```python
from build123d import *

# Parameters (mm, degrees)
ESBO_O1_W                                            = 10
ESBO_O1_H                                            = 11.5
RESSALTO_EXTRUS_O1_DEPTH                             = 9
ESBO_O2_W                                            = 4
ESBO_O2_H                                            = 0.85
CORTE_EXTRUS_O1_DEPTH                                = 10
ESBO_O3_W                                            = 3
ESBO_O3_H                                            = 1.6
RESSALTO_EXTRUS_O2_DEPTH                             = 1
ESBO_O4_W                                            = 3
ESBO_O4_H                                            = 1.6
RESSALTO_EXTRUS_O3_DEPTH                             = 1
ESBO_O5_W                                            = 4
ESBO_O5_H                                            = 1.5
CORTE_EXTRUS_O2_DEPTH                                = 11
ESBO_O6_W                                            = 1.5
ESBO_O6_H                                            = 1
RESSALTO_EXTRUS_O4_DEPTH                             = 1
ESBO_O7_W                                            = 1.5
ESBO_O7_H                                            = 1.5
CORTE_EXTRUS_O3_DEPTH                                = 6
ESBO_O8_W                                            = 1.5
ESBO_O8_H                                            = 1
RESSALTO_EXTRUS_O5_DEPTH                             = 1
ESBO_O9_W                                            = 1.5
ESBO_O9_H                                            = 1.5
CORTE_EXTRUS_O4_DEPTH                                = 6
ESBO_O10_W                                           = 1.5
ESBO_O10_H                                           = 1.5
RESSALTO_EXTRUS_O6_DEPTH                             = 1.5
ESBO_O11_W                                           = 1.5
ESBO_O11_H                                           = 1.5
RESSALTO_EXTRUS_O7_DEPTH                             = 1.5
ESBO_O12_W                                           = 9.5
ESBO_O12_H                                           = 4.15
REBAIXO_PARA_PARAFUSO_DE_M_QUINA_DE_CABE_D           = 3.3
REBAIXO_PARA_PARAFUSO_DE_M_QUINA_DE_CABE_DEPTH       = 9.5
REBAIXO_PARA_PARAFUSO_DE_M_QUINA_DE_CABE_CBORE_D     = 6
REBAIXO_PARA_PARAFUSO_DE_M_QUINA_DE_CABE_CBORE_DEPTH = 0.375
FILETE1_R                                            = 1
RESSALTO_EXTRUS_O9_DEPTH                             = 0.2


with BuildPart() as part:
    # Esboço1 → Ressalto-extrusão1 (new body)
    with BuildSketch(Plane(origin=(10, 0, 0), x_dir=(0, 0, -1), z_dir=(1, 0, 0))):
        with Locations((0, -0.75)):
            Rectangle(ESBO_O1_W, ESBO_O1_H)
    extrude(amount=-RESSALTO_EXTRUS_O1_DEPTH)

    # Esboço2 → Corte-extrusão1 (cut, through all)
    with BuildSketch(Plane(origin=(10, 0, 0), x_dir=(0, 0, -1), z_dir=(1, 0, 0))):
        with Locations((0, 4.575)):
            Rectangle(ESBO_O2_W, ESBO_O2_H)
    extrude(amount=-CORTE_EXTRUS_O1_DEPTH, mode=Mode.SUBTRACT)

    # Esboço3 → Ressalto-extrusão2 (add)
    with BuildSketch(Plane.ZY.offset(-1)):
        with Locations((3.5, 4.2)):
            Rectangle(ESBO_O3_W, ESBO_O3_H)
    extrude(amount=RESSALTO_EXTRUS_O2_DEPTH)

    # Esboço4 → Ressalto-extrusão3 (add)
    with BuildSketch(Plane.ZY.offset(-1)):
        with Locations((-3.5, 4.2)):
            Rectangle(ESBO_O4_W, ESBO_O4_H)
    extrude(amount=RESSALTO_EXTRUS_O3_DEPTH)

    # Esboço5 → Corte-extrusão2 (cut, through all)
    with BuildSketch(Plane(origin=(10, 0, 0), x_dir=(0, 0, -1), z_dir=(1, 0, 0))):
        with Locations((0, -5.75)):
            Rectangle(ESBO_O5_W, ESBO_O5_H)
    extrude(amount=-CORTE_EXTRUS_O2_DEPTH, mode=Mode.SUBTRACT)

    # Esboço6 → Ressalto-extrusão4 (add)
    with BuildSketch(Plane.ZY.offset(-1)):
        with Locations((2.75, -6)):
            Rectangle(ESBO_O6_W, ESBO_O6_H)
    extrude(amount=RESSALTO_EXTRUS_O4_DEPTH)

    # Esboço7 → Corte-extrusão3 (cut)
    with BuildSketch(Plane.ZY.offset(-1)):
        with Locations((4.25, -5.75)):
            Rectangle(ESBO_O7_W, ESBO_O7_H)
    extrude(amount=-CORTE_EXTRUS_O3_DEPTH, mode=Mode.SUBTRACT)

    # Esboço8 → Ressalto-extrusão5 (add)
    with BuildSketch(Plane.ZY.offset(-1)):
        with Locations((-2.75, -6)):
            Rectangle(ESBO_O8_W, ESBO_O8_H)
    extrude(amount=RESSALTO_EXTRUS_O5_DEPTH)

    # Esboço9 → Corte-extrusão4 (cut)
    with BuildSketch(Plane.ZY.offset(-1)):
        with Locations((-4.25, -5.75)):
            Rectangle(ESBO_O9_W, ESBO_O9_H)
    extrude(amount=-CORTE_EXTRUS_O4_DEPTH, mode=Mode.SUBTRACT)

    # Esboço10 → Ressalto-extrusão6 (add)
    with BuildSketch(Plane.XZ.offset(6.5)):
        with Locations((9.25, 4.25)):
            Rectangle(ESBO_O10_W, ESBO_O10_H)
    extrude(amount=RESSALTO_EXTRUS_O6_DEPTH)

    # Esboço11 → Ressalto-extrusão7 (add)
    with BuildSketch(Plane.XZ.offset(6.5)):
        with Locations((9.25, -4.25)):
            Rectangle(ESBO_O11_W, ESBO_O11_H)
    extrude(amount=RESSALTO_EXTRUS_O7_DEPTH)

    # Esboço12 → Revolução1 (revolve)
    with BuildSketch(Plane.XY):
        with Locations((14.75, 2.075)):
            Rectangle(ESBO_O12_W, ESBO_O12_H)
    revolve(axis=Axis((10, 0, 0), (1, 0, 0)))

    # Rebaixo para parafuso de máquina de cabeça sextavada de M31
    with Locations(Plane(origin=(19.5, 0, 0), x_dir=(0, 0, -1), z_dir=(1, 0, 0))):
        with Locations((0, 0)):
            CounterBoreHole(REBAIXO_PARA_PARAFUSO_DE_M_QUINA_DE_CABE_D / 2, REBAIXO_PARA_PARAFUSO_DE_M_QUINA_DE_CABE_CBORE_D / 2, REBAIXO_PARA_PARAFUSO_DE_M_QUINA_DE_CABE_CBORE_DEPTH, depth=REBAIXO_PARA_PARAFUSO_DE_M_QUINA_DE_CABE_DEPTH)

    # Filete1
    filete1_edges = [part.edges().sort_by_distance(p)[0] for p in [
        (19.5, -4.15, 0),
    ]]
    fillet(filete1_edges, radius=FILETE1_R)

    # Esboço16 → Ressalto-extrusão9 (add, symmetric)
    with BuildSketch(Plane(origin=(0, 0, 0), x_dir=(-1, 0, 0), z_dir=(0, 0, -1))):
        with BuildLine():
            Line((-2, -5), (-2, -9.5))
            ThreePointArc((-2, -9.5), (-1.569549144, -9.99513929), (-1.019348334, -9.637746055))
            Line((-1.019348334, -9.637746055), (-0.549999999, -8))
            Line((-0.549999999, -8), (-0.8, -7.928354531))
            Line((-0.8, -7.928354531), (-0.8, 3.5))
            Line((-0.8, 3.5), (-1, 3.5))
            Line((-1, 3.5), (-2, -5))
        make_face()
    extrude(amount=RESSALTO_EXTRUS_O9_DEPTH, both=True)


solid = part.part
```
The model under review builds one solid part; all positions refer to its coordinate system, in mm. A direction names the side the tool comes from. Round coordinates to 2 decimals unless told otherwise and drop trailing zeros. Order: outer loops, then holes, each group sorted by start corner. A loop starts at its lowest first (then second) coordinate and runs counter-clockwise, first axis right, second up.
Item 1: Draft analysis for pull direction Y (two halves, no side actions). For faces 5 (the flat face through (9, -8, -4)), 6 (the flat face through (0.5, -5.5, 2.7)), 7 (the flat face through (9, -7, 3.5)), state which applies: released by +Y, released by -Y, zero draft, split by the parting line, or undercut.
Working result:
face 5: released by -Y
face 6: undercut
face 7: zero draft
Item 2: Add section A-A, the plane y = -6. State the section outline as (x, z) points.
Working result:
outline: (0, -3.5) - (7, -3.5) - (7, -5) - (10, -5) - (10, -2) - (0, -2) - close; (0, 2) - (10, 2) - (10, 5) - (7, 5) - (7, 3.5) - (0, 3.5) - close; (0.8, -0.2) - (2, -0.2) - (2, 0.2) - (0.8, 0.2) - close
Item 3: For pin 1 (1.2 mm diameter, centred on x = 5, y = -6, fed in from +Z); pin 2 (1.6 mm diameter, centred on x = 9, z = -4, fed in from -Y); pin 3 (1.5 mm diameter, centred on x = 13, z = 1, fed in from -Y), all flat-tipped, find the tip position at first contact; note any pin that passes through.
Working result:
pin 1: stops at z = 3.5
pin 2: stops at y = -8
pin 3: stops at y = -4.14
Item 4: Add section C-C, the plane x = 12.75. State the section outline as (y, z) points, and give its area (3 significant figures).
Working result:
outline: circle Ø8.3 at (0, 0); hole circle Ø3.3 at (0, 0)
area: 45.6 mm2
Item 5: To check wall thickness, follow probe 1 along Z at (x, y) = (8, -6.25); probe 2 along X at (y, z) = (2.75, 1.5); probe 3 along Y at (x, z) = (4.25, -4). State the ranges of each line that lie inside material, in increasing order.
Working result:
probe 1: z = -5 to -2, 2 to 5
probe 2: x = 1 to 19.5
probe 3: y = -5 to 5
Item 6: Add section B-B, the plane y = -4.5. State the section outline as (x, z) points, and give its area (3 significant figures).
Working result:
outline: (0.8, -0.2) - (1, -0.2) - (1, -5) - (10, -5) - (10, 5) - (1, 5) - (1, 0.2) - (0.8, 0.2) - close
area: 90.1 mm2
Item 7: Add section D-D, the plane y = 0. State the section outline as (x, z) points (3 decimals), and give its area (3 significant figures).
Working result:
outline: (0.8, -0.2) - (1, -0.2) - (1, -5) - (10, -5) - (10, -4.15) - (18.5, -4.15) arc R1 ccw to (19.5, -3.15) - (19.5, -3) - (19.125, -3) - (19.125, -1.65) - (10, -1.65) - (10, 1.65) - (19.125, 1.65) - (19.125, 3) - (19.5, 3) - (19.5, 3.15) arc R1 ccw to (18.5, 4.15) - (10, 4.15) - (10, 5) - (1, 5) - (1, 0.2) - (0.8, 0.2) - close
area: 136 mm2
Item 8: Machinability: for faces 1 (the flat face through (4, -6, -3.5)), 2 (the cylindrical face through (19.3, 0.1, 3)), 3 (the flat face through (8.5, -7, -4)), 4 (the flat face through (9, -7, -3.5)), which of the approach directions +Z, -Z, +X, -X, +Y, -Y give a long, thin tool a straight path to every point of the face, cutting with its end or side? Answer none if there is none.
Working result:
face 1: -Z, -X, -Y
face 2: +X
face 3: +Z, -Z, -X, -Y
face 4: +X, -X, -Y
